Work out the finished part from the listing and answer in its coordinate system (mm). A direction names the side the tool comes from. Round coordinates to 2 decimals unless told otherwise and drop trailing zeros. Write each loop counter-clockwise with the first axis right and the second up, starting at its lowest first coordinate (ties: lowest second). Pieces come first, ordered by that corner, then holes. Notation, with made-up numbers: (39, -18.75) - (75, -18.75) arc R14 ccw to (75, -6.75) - close; hole circle Ø4 at (-14, 11.5). An arc over 180 degrees is marked (long way). Write item = value, one per line. Start each with the question number.
from build123d import *

# Parameters (mm, degrees)
SKETCH1_W     = 7.5
SKETCH1_H     = 7
CHAMFER1_SIZE = 0.1


with BuildPart() as part:
    # Sketch1 → Revolve1 (revolve)
    with BuildSketch(Plane(origin=(0, 0, 0), x_dir=(0, 0, -1), z_dir=(1, 0, 0))):
        with Locations((33.75, 0)):
            Rectangle(SKETCH1_W, SKETCH1_H)
    revolve(axis=Axis((0, 3.5, 0), (0, -1, 0)))

    # Sketch3 → Cut-Revolve2 (revolve, cut)
    with BuildSketch(Plane(origin=(0, 0, 0), x_dir=(0, 0, -1), z_dir=(1, 0, 0))):
        Polygon((35.3, 3.3), (35.5, 3.1), (35.5, 3.5), (32, 3.5), (32, 3.1), (32.2, 3.3), align=None)
    cut_revolve2 = revolve(axis=Axis((0, 3.5, 0), (0, -1, 0)), mode=Mode.SUBTRACT)

    # Mirror1: Cut-Revolve2 across plane
    add(cut_revolve2.mirror(Plane.ZX), mode=Mode.SUBTRACT)

    # Chamfer1
    chamfer1_edges = [part.edges().sort_by_distance(p)[0] for p in [
        (0, 3.5, 35.5),
        (0, 3.5, 32),
        (0, -3.5, 35.5),
        (0, -3.5, 32),
        (0, 3.5, 37.5),
        (0, -3.5, 37.5),
        (0, -3.5, 30),
        (0, 3.5, 30),
    ]]
    chamfer(chamfer1_edges, length=CHAMFER1_SIZE)


solid = part.part
1. Each of these flat-tipped pins is pushed along its axis until it touches: pin 1 (1.5 mm diameter, centred on y = 1, z = -10, fed in from +X); pin 2 (1 mm diameter, centred on y = -2, z = -26.5, fed in from -X); pin 3 (4 mm diameter, centred on y = 2, z = 20.5, fed in from +X). Where does it stop, or does it pass through?
2. Find section A-A on y = 1.25. Give the vertices of the cut face in (x, z).
3. Which of the six approach directions +Z, -Z, +X, -X, +Y, -Y give full straight-line access (tool end or side, diameter ignored) to faces 1 (the face through (-29, -3.3, 16)), 2 (the face through (-14, -3.5, 33))?
4. Consider line 1 (X direction, y = -1.25, z = 0); line 2 (X direction, y = 0.5, z = -5); line 3 (Y direction, x = 20, z = 27). Determine where each line is inside the solid, lowest interval first.
Answer key:
q1.pin_1 = 36.34
q1.pin_2 = -27.02
q1.pin_3 = 32.62
q2.outline = circle Ø75 at (0, 0); hole circle Ø60 at (0, 0)
q3.face_1 = -Y
q3.face_2 = +Z, -Z, +X, -X, -Y
q4.line_1 = -37.5 to -30, 30 to 37.5
q4.line_2 = -37.17 to -29.58, 29.58 to 37.17
q4.line_3 = -3.3 to 3.3
